Build history of the part. All positions in model axes, mm. Face numbers are marked on the shaded views. A direction names the side the tool comes from. Round coordinates to 2 decimals unless told otherwise and drop trailing zeros. Write each loop counter-clockwise with the first axis right and the second up, starting at its lowest first coordinate (ties: lowest second). Pieces come first, ordered by that corner, then holes. Notation, with made-up numbers: (57, -27.75) - (83, -27.75) arc R35 cw to (83, 8.25) - close; hole circle Ø6 at (26, 78.25). An arc over 180 degrees is marked (long way). Answer as a JSON object with one key per item and string values. Group by question number.
Item 1: Two-plate mould, pull along Z, no slides. Class the marked faces 5, 6 and 7: +Z half, -Z half, draft (parallel to the pull), parting line (faces both ways), or undercut.
Item 2: Which spindle directions (+Z, -Z, +X, -X, +Y, -Y) get a long thin tool onto all of the face, cutting with end or side? Do the marked faces 1, 2, 3 and 4. Say none if no direction does.
Item 3: Slice it at C-C, the plane z = 0. List the corners of the cut face in (x, y), then the cut area to 3 significant figures.
Item 4: Slice it at B-B, the plane y = 46.5. List the corners of the cut face in (x, z).
Item 5: Slice it at D-D, the plane z = 14. List the corners of the cut face in (x, y).
Item 6: Slice it at A-A, the plane x = 0. List the corners of the cut face in (y, z).
Item 7: Flat gauge pins, fed straight in: pin 1 (1 mm diameter, centred on x = 20, z = 23.5, fed in from +Y); pin 2 (8 mm diameter, centred on x = -33, y = 24.5, fed in from -Z); pin 3 (2.5 mm diameter, centred on x = 0.5, z = 34.5, fed in from -Y); pin 4 (5.5 mm diameter, centred on y = 33.5, z = 33.5, fed in from +X). Where does each tip first touch, or does it go through?
Item 8: Probe line 1 (Z direction, x = 8, y = 23); line 2 (X direction, y = 34.5, z = 34.85); line 3 (Z direction, x = 17, y = 49.5). List the from-to ranges inside material, lowest first. Write a range as from..to.
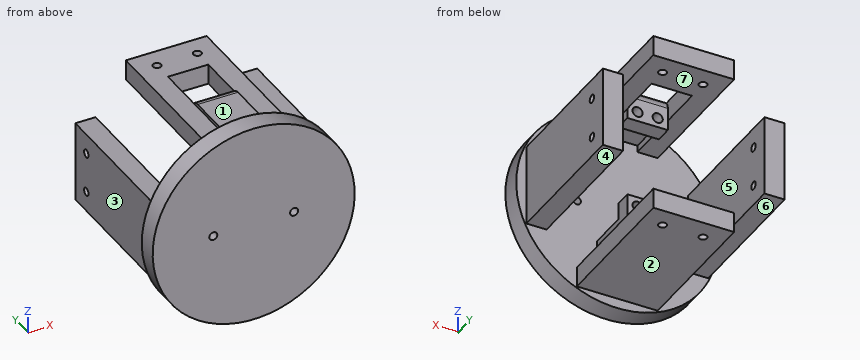
from build123d import *

# Parameters (mm, degrees)
SKETCH1_R                = 50
BOSS_EXTRUDE1_DEPTH      = 10
SKETCH2_W                = 20
SKETCH2_H                = 8.2
BOSS_EXTRUDE2_DEPTH      = 27.8
SKETCH3_W                = 20
SKETCH3_H                = 8.2
BOSS_EXTRUDE3_DEPTH      = 8.2
SKETCH4_W                = 20
SKETCH4_H                = 8.199243263
BOSS_EXTRUDE4_DEPTH      = 8.2
FILLET1_R                = 5
SKETCH7_R                = 2.5
CUT_EXTRUDE1_DEPTH       = 9
SKETCH5_W                = 10
SKETCH5_H                = 10
BOSS_EXTRUDE5_DEPTH      = 70
BOSS_EXTRUDE6_REACH      = 113.803
SKETCH8_W                = 10
SKETCH8_H                = 20
F_4_0_4_DIAMETER_HOLE1_D = 4
F_4_0_4_DIAMETER_HOLE2_D = 4
F_4_0_4_DIAMETER_HOLE3_D = 4


with BuildPart() as part:
    # Sketch1 → Boss-Extrude1 (new body)
    with BuildSketch(Plane(origin=(0, 0, 0), x_dir=(1, 0, 0), z_dir=(0, 1, 0))):
        with Locations(Location((0, 0, 0), (0, 0, 270))):
            Circle(SKETCH1_R)
    extrude(amount=BOSS_EXTRUDE1_DEPTH)

    # Sketch2 → Boss-Extrude2 (add)
    with BuildSketch(Plane(origin=(0, 10, 0), x_dir=(1, 0, 0), z_dir=(0, 1, 0))):
        with Locations((0, -42.4)):
            Rectangle(SKETCH2_W, SKETCH2_H)
        with Locations((0, 22.2)):
            Rectangle(SKETCH2_W, SKETCH2_H)
    extrude(amount=BOSS_EXTRUDE2_DEPTH)

    # Sketch3 → Boss-Extrude3 (add)
    with BuildSketch(Plane(origin=(0, 0, 38.3), x_dir=(-1, 0, 0), z_dir=(0, 0, -1))):
        with Locations((0, 33.7)):
            Rectangle(SKETCH3_W, SKETCH3_H)
    extrude(amount=BOSS_EXTRUDE3_DEPTH)

    # Sketch4 → Boss-Extrude4 (add)
    with BuildSketch(Plane.XY.offset(-18.1)):
        with Locations((0, 33.700378369)):
            Rectangle(SKETCH4_W, SKETCH4_H)
    extrude(amount=BOSS_EXTRUDE4_DEPTH)

    # Fillet1
    fillet1_edges = [part.edges().sort_by_distance(p)[0] for p in [
        (0, 37.8, -26.3),
        (0, 37.8, 46.5),
    ]]
    fillet(fillet1_edges, radius=FILLET1_R)

    # Sketch7 → Cut-Extrude1 (cut)
    with BuildSketch(Plane(origin=(0, 37.8, 0), x_dir=(1, 0, 0), z_dir=(0, 1, 0))):
        with Locations(Location((5, 14.65, 0), (0, 0, 270))):
            Circle(SKETCH7_R)
        with Locations(Location((-5, 14.65, 0), (0, 0, 270))):
            Circle(SKETCH7_R)
        with Locations(Location((-5, -34.85, 0), (0, 0, 270))):
            Circle(SKETCH7_R)
        with Locations(Location((5, -34.85, 0), (0, 0, 270))):
            Circle(SKETCH7_R)
    extrude(amount=-CUT_EXTRUDE1_DEPTH, mode=Mode.SUBTRACT)

    # Sketch5 → Boss-Extrude5 (add)
    with BuildSketch(Plane(origin=(0, 10, 0), x_dir=(1, 0, 0), z_dir=(0, 1, 0))):
        Polygon((35, 0), (35, 20), (45, 20), (45, -20), (35, -20), align=None)
        Polygon((-45, -20), (-35, -20), (-35, 0), (-35, 20), (-45, 20), align=None)
        with Locations((-15, -40)):
            Rectangle(SKETCH5_W, SKETCH5_H)
        with Locations((15, -40)):
            Rectangle(SKETCH5_W, SKETCH5_H)
        Polygon((-20, 35), (-20, 45), (20, 45), (20, 35), (0, 35), align=None)
    extrude(amount=BOSS_EXTRUDE5_DEPTH)

    # Sketch8 → Boss-Extrude6 (add, up to next)
    with BuildSketch(Plane.ZY.offset(-10), mode=Mode.PRIVATE) as boss_extrude6_sk1:
        with Locations((40, 70)):
            Rectangle(SKETCH8_W, SKETCH8_H)
    boss_extrude6_tool1 = extrude(boss_extrude6_sk1.sketch, amount=BOSS_EXTRUDE6_REACH, mode=Mode.PRIVATE) - part.part
    add(boss_extrude6_tool1.solids().sort_by_distance((10, 70, 40))[0])

    # Ø4.0 (4) Diameter Hole1 (through all)
    with Locations(Plane.XY.offset(45)):
        with Locations((-10, 70), (10, 70)):
            Hole(F_4_0_4_DIAMETER_HOLE1_D / 2)

    # Ø4.0 (4) Diameter Hole2 (through all)
    with Locations(Plane(origin=(45, 0, 0), x_dir=(0, 0, -1), z_dir=(1, 0, 0))):
        with Locations((-10, 70), (10, 70)):
            Hole(F_4_0_4_DIAMETER_HOLE2_D / 2)

    # Ø4.0 (4) Diameter Hole3 (through all)
    with Locations(Plane(origin=(0, 10, 0), x_dir=(1, 0, 0), z_dir=(0, 1, 0))):
        with Locations((-20, 0), (20, 0)):
            Hole(F_4_0_4_DIAMETER_HOLE3_D / 2)


solid = part.part
Geometry says:
{
 "1": {"face 5": "draft", "face 6": "-Z half", "face 7": "undercut"},
 "2": {"face 1": "+Z, +X, -X, +Y", "face 2": "-Z, +X, -X, +Y", "face 3": "+Z, -Z, -X, +Y", "face 4": "-Z, +X, +Y"},
 "3": {"outline": "(-50, 0) - (-22, 0) - (-22, 10) - (-35, 10) - (-35, 80) - (-45, 80) - (-45, 10) - (-50, 10) - close; (-18, 0) - (18, 0) - (18, 10) - (-18, 10) - close; (22, 0) - (50, 0) - (50, 10) - (45, 10) - (45, 80) - (35, 80) - (35, 10) - (22, 10) - close", "area": "2,320 mm^2"},
 "4": {"outline": "(-45, -20) - (-35, -20) - (-35, 20) - (-45, 20) - close; (-20, -45) - (20, -45) - (20, -35) - (-20, -35) - close; (-20, 35) - (-10, 35) - (-10, 45) - (-20, 45) - close; (10, 35) - (20, 35) - (20, 45) - (10, 45) - close; (35, -20) - (45, -20) - (45, 20) - (35, 20) - close"},
 "5": {"outline": "(-48, 0) - (48, 0) - (48, 10) - (45, 10) - (45, 80) - (35, 80) - (35, 10) - (-35, 10) - (-35, 80) - (-45, 80) - (-45, 10) - (-48, 10) - close"},
 "6": {"outline": "(0, -50) - (10, -50) - (10, -45) - (80, -45) - (80, -35) - (10, -35) - (10, -26.3) - (32.8, -26.3) arc R5 ccw to (37.8, -21.3) - (37.8, -9.9) - (29.6, -9.9) - (29.6, -18.1) - (10, -18.1) - (10, 38.3) - (29.6, 38.3) - (29.6, 30.1) - (37.8, 30.1) - (37.8, 41.5) arc R5 ccw to (32.8, 46.5) - (10, 46.5) - (10, 50) - (0, 50) - close; (60, 35) - (80, 35) - (80, 45) - (60, 45) - close"},
 "7": {"pin 1": "stops at y = 10", "pin 2": "stops at z = -20", "pin 3": "stops at y = 0", "pin 4": "stops at x = 20"},
 "8": {"line 1": "z = -45..-35, -26.3..-18.1, 38.3..46.5", "line 2": "x = -10..-7.5, -2.5..2.5, 7.5..10", "line 3": "z = -45..-35, 35..45"}
}
